CAD build for the part. Positions are in the model's coordinates, mm. A direction names the side the tool comes from. Coordinates: 2 decimals unless noted, no trailing zeros. Loops run counter-clockwise (first coordinate to the right, second up) from the corner with the lowest first, then second, coordinate; pieces in that order, holes last. Notation, with made-up numbers: (18, 78.25) -> (54, 78.25) arc R7 cw to (54, 83.25) -> close; hole circle Ø10 at (-32, 58). An arc over 180 degrees is marked (long way). Write each question's results on one line, items separated by ' | '.
from build123d import *

# Parameters (mm, degrees)
SKETCH1_W           = 70
SKETCH1_H           = 40
BOSS_EXTRUDE1_DEPTH = 3
SKETCH2_R           = 14.255
CUT_EXTRUDE1_DEPTH  = 3


with BuildPart() as part:
    # Sketch1 → Boss-Extrude1 (new body)
    with BuildSketch(Plane(origin=(0, 0, 0), x_dir=(1, 0, 0), z_dir=(0, 1, 0))):
        with Locations((35, 20)):
            Rectangle(SKETCH1_W, SKETCH1_H)
    extrude(amount=BOSS_EXTRUDE1_DEPTH)

    # Sketch2 → Cut-Extrude1 (cut)
    with BuildSketch(Plane(origin=(0, 3, 0), x_dir=(1, 0, 0), z_dir=(0, 1, 0))):
        with Locations((35.9375, 20)):
            Circle(SKETCH2_R)
        with BuildLine():
            Line((12.625, 35), (12.625, 5))
            ThreePointArc((12.625, 5), (10, 2.375), (7.375, 5))
            Line((7.375, 5), (7.375, 35))
            ThreePointArc((7.375, 35), (10, 37.625), (12.625, 35))
        make_face()
        with BuildLine():
            Line((64.5, 35), (64.5, 5))
            ThreePointArc((64.5, 5), (61.875, 2.375), (59.25, 5))
            Line((59.25, 5), (59.25, 35))
            ThreePointArc((59.25, 35), (61.875, 37.625), (64.5, 35))
        make_face()
    extrude(amount=-CUT_EXTRUDE1_DEPTH, mode=Mode.SUBTRACT)


solid = part.part
1) Slice it at A-A (z = -20). Count the separate pieces of the cut face and the enclosed holes in it, then the cut area to 3 significant figures.
Outcome:
separate pieces: 4 | enclosed holes: 0 | area: 93.0 mm^2
2) Which spindle directions (+Z, -Z, +X, -X, +Y, -Y) get a long thin tool onto all of the face, cutting with end or side? Do faces 1 (the cylindrical face through (10.058, 1.521, -2.376)), 2 (the flat face through (50, 0, -25)). Say none if no direction does.
Outcome:
face 1: +Y, -Y | face 2: +Z, -Z, +X, -X, -Y
3) Slice it at D-D (z = -8.5). Write the cut outline in (x, y) (3 decimals).
Outcome:
outline: (0, 0) -> (7.375, 0) -> (7.375, 3) -> (0, 3) -> close; (12.625, 0) -> (27.514, 0) -> (27.514, 3) -> (12.625, 3) -> close; (44.361, 0) -> (59.25, 0) -> (59.25, 3) -> (44.361, 3) -> close; (64.5, 0) -> (70, 0) -> (70, 3) -> (64.5, 3) -> close
4) Two-plate mould, pull along X, no slides. Class faces 3 (the flat face through (35, 1, -40)), 4 (the flat face through (0, 1, -20)), 5 (the cylindrical face through (61.817, 1.521, -37.624)), 6 (the cylindrical face through (49.105, 1.521, -14.54)): pulls with the +X half, pulls with the -X half, needs draft (parallel to the pull), parting line crosses it, or undercut.
Outcome:
face 3: needs draft | face 4: pulls with the -X half | face 5: undercut | face 6: undercut
5) Slice it at B-B (x = 10). Write the cut outline in (y, z) (3 decimals).
Outcome:
outline: (0, -40) -> (3, -40) -> (3, -37.625) -> (0, -37.625) -> close; (0, -2.375) -> (3, -2.375) -> (3, 0) -> (0, 0) -> close
6) Drill centre lines: L1, parallel to Z at x = 10, y = 1.25 (3 decimals); L2, parallel to X at y = 2.8, z = -10.5 (3 decimals); L3, parallel to X at y = 1.2, z = -24 (3 decimals). Where is each one in solid material? Low to high. Write a range as from..to.
Outcome:
L1: z = -40..-37.625, -2.375..0 | L2: x = 0..7.375, 12.625..25.309, 46.566..59.25, 64.5..70 | L3: x = 0..7.375, 12.625..22.255, 49.62..59.25, 64.5..70
7) Pin check, flat tip, straight feed: pin 1 (3 mm diameter, centred on x = 15.5, z = -22, fed in from -Y). Stop position of the tip, or through.
Outcome:
pin 1: stops at y = 0
